Part model, mm, in its own coordinate system. A direction names the side the tool comes from. Round coordinates to 2 decimals unless told otherwise and drop trailing zeros. Order: outer loops, then holes, each group sorted by start corner. A loop starts at its lowest first (then second) coordinate and runs counter-clockwise, first axis right, second up. Notation, with made-up numbers: M 4.5,-16.5 L 44.5,-16.5 A21 ccw 44.5,16.5 Z; hole C 78,70 d6. An arc over 180 degrees is marked long. Write each question's results on one line, items separated by ' | '. Start each with the question number.
1. Which spindle directions (+Z, -Z, +X, -X, +Y, -Y) get a long thin tool onto all of the face, cutting with end or side? Do faces 4 (the face through (4, 67, 5)), 5 (the face through (3.7, -30.4, 25)). Say none if no direction does.
2. Band-saw the part on B-B, the plane x = 31.5. List the corners of the cut face in (y, z).
3. Two-plate mould, pull along X, no slides. Class faces 1 (the face through (-0.3, -30.4, 0)), 2 (the face through (-42.64, -15.594, 12.325)), 3 (the face through (0, 68, 15)): +X half, -X half, draft (parallel to the pull), parting line (faces both ways), or undercut.
4. Drop flat-ended pins along their axis: pin 1 Ø4 at (x, z) = (-25, 10.5) entering from +Y; pin 2 Ø1 at (y, z) = (32, 12.5) entering from +X; pin 3 Ø2 at (x, z) = (16.5, 13) entering from -Y. Give the stop position or say it passes through.
5. Probe L1, parallel to Y at x = 1.5, z = 6; L2, parallel to X at y = 20.5, z = 5; L3, parallel to X at y = 19, z = 7.25. List the from-to ranges inside material, lowest first. Write a range as [from, to].
6. Band-saw the part on C-C, the plane z = 9. List the corners of the cut face in (x, y), then the cut area to 3 significant figures.
7. Band-saw the part on A-A, the plane y = 25. List the corners of the cut face in (x, z).
```python
from build123d import *

# Parameters (mm, degrees)
F0_R     = 53.731796632
F0_R_2   = 47.3494506103
F1_DEPTH = 25
F3_DEPTH = 20


with BuildPart() as f1:
    # F0 (on Top) → F1 (new body)
    with BuildSketch(Plane.XY):
        with Locations((0, 17.1008221805)):
            Circle(F0_R)
        with Locations((0, 17.1008221805)):
            Circle(F0_R_2, mode=Mode.SUBTRACT)
    extrude(amount=F1_DEPTH)

    # F2 (on face) → F3 (cut)
    with BuildSketch(Plane.XY.offset(25)):
        with BuildLine():
            Line((0, 70.8326188125), (0, 64.4502727909))
            ThreePointArc((0, 64.4502727909), (4.1053363789, 64.2719646971), (8.1797530875, 63.7383833574))
            Line((8.1797530875, 63.7383833574), (8.1797530875, 70.2063549312))
            ThreePointArc((8.1797530875, 70.2063549312), (4.1018461399, 70.6758240708), (0, 70.8326188125))
        make_face()
    extrude(amount=-F3_DEPTH, mode=Mode.SUBTRACT)


solid = f1.part
```
Solution:
1) face 4: +Z, +Y | face 5: +Z, +X, -X, +Y, -Y
2) outline: M -26.43,0 L -18.25,0 L -18.25,25 L -26.43,25 Z; M 52.45,0 L 60.63,0 L 60.63,25 L 52.45,25 Z
3) face 1: draft | face 2: parting line | face 3: undercut
4) pin 1: y = 65.66 | pin 2: x = 51.77 | pin 3: y = -34.35
5) L1: [-36.61, -30.22] | L2: [-53.62, -47.23], [47.23, 53.62] | L3: [-53.7, -47.31], [47.31, 53.7]
6) outline: M 0,64.45 L 0,70.83 A53.73 ccw long 8.18,70.21 L 8.18,63.74 A47.35 cw long Z | area: 1,970 mm^2
7) outline: M -53.15,0 L -46.69,0 L -46.69,25 L -53.15,25 Z; M 46.69,0 L 53.15,0 L 53.15,25 L 46.69,25 Z
